Can you work these out from the model? Positions are in its coordinate system, mm. A direction names the side the tool comes from. Give positions to 0.01 mm unless a question says otherwise; leave off trailing zeros. Loops run counter-clockwise (first coordinate to the right, second up) from the corner with the lowest first, then second, coordinate; pieces in that order, holes last.
from build123d import *

# Parameters (mm, degrees)
SKETCH1_R           = 2.794
BOSS_EXTRUDE1_DEPTH = 5.08
SKETCH3_W           = 25.4
SKETCH3_H           = 11.43
BOSS_EXTRUDE2_DEPTH = 45.72
SKETCH4_W           = 22.096687199
SKETCH4_H           = 11.43
BOSS_EXTRUDE3_DEPTH = 12.7
BOSS_EXTRUDE5_DEPTH = 11.43
SKETCH7_W           = 18.793374398
SKETCH7_H           = 33.02
CUT_EXTRUDE3_DEPTH  = 12.7


with BuildPart() as part:
    # Sketch1 → Boss-Extrude1 (new body)
    with BuildSketch(Plane.XY):
        Polygon((-57.15, 2.54), (-57.15, -2.54), (-57.15, -5.715), (57.15, -5.715), (57.15, -2.54), (57.15, 2.54), (57.15, 5.715), (-57.15, 5.715), align=None)
        with Locations((50.8, 0)):
            Circle(SKETCH1_R, mode=Mode.SUBTRACT)
        with Locations((-50.8, 0)):
            Circle(SKETCH1_R, mode=Mode.SUBTRACT)
    extrude(amount=BOSS_EXTRUDE1_DEPTH)

    # Sketch3 → Boss-Extrude2 (add)
    with BuildSketch(Plane.XY.offset(5.08)):
        Rectangle(SKETCH3_W, SKETCH3_H)
    extrude(amount=BOSS_EXTRUDE2_DEPTH)

    # Sketch4 → Boss-Extrude3 (add)
    with BuildSketch(Plane.XY.offset(50.8)):
        with Locations((23.7483436, 0)):
            Rectangle(SKETCH4_W, SKETCH4_H)
        with Locations((-23.7483436, 0)):
            Rectangle(SKETCH4_W, SKETCH4_H)
    extrude(amount=-BOSS_EXTRUDE3_DEPTH)

    # Sketch5 → Boss-Extrude5 (add)
    with BuildSketch(Plane.XZ.offset(5.715)):
        Polygon((-44.45, 5.08), (-12.7, 5.08), (-12.7, 38.1), (-21.519444444, 38.1), align=None)
        Polygon((12.7, 38.1), (12.7, 5.08), (44.45, 5.08), (21.519444444, 38.1), align=None)
    extrude(amount=-BOSS_EXTRUDE5_DEPTH)

    # Sketch7 → Cut-Extrude3 (cut)
    with BuildSketch(Plane.XZ.offset(5.715)):
        with Locations((0, 21.59)):
            Rectangle(SKETCH7_W, SKETCH7_H)
    extrude(amount=-CUT_EXTRUDE3_DEPTH, mode=Mode.SUBTRACT)


solid = part.part
(1) Which directions (+Z, -Z, +X, -X, +Y, -Y) give clear straight access to the entire face, cutting with the end or side of a thin tool? Please do faces 1 (the flat face through (-9.397, 0, 21)), 2 (the flat face through (49, 3, 5.08)), 3 (the flat face through (-32.824, -0.08, 21.821)).
Returned:
face 1: +Y, -Y
face 2: +Z, +X, +Y, -Y
face 3: -X, +Y, -Y
(2) Will these pins go through, and if not, where does the flat tip stop? P1, Ø5.5, axis at x = -52, y = -1, coming from the +Z side; P2, Ø5, axis at x = 12.5, y = -3, coming from the -Z side; P3, Ø3.5, axis at y = -1.5, z = 45.5, coming from the +X side; P4, Ø4, axis at y = 3.5, z = 33, coming from the +X side.
Returned:
P1: stops at z = 5.08
P2: stops at z = 0
P3: stops at x = 34.8
P4: stops at x = 26.45
(3) Suppose I cut it at B-B on y = 0. List the corners of the cut face in (x, z) for me.
Returned:
outline: (-57.15, 0) - (-53.59, 0) - (-53.59, 5.08) - (-57.15, 5.08) - close; (-48.01, 0) - (48.01, 0) - (48.01, 5.08) - (44.45, 5.08) - (21.52, 38.1) - (34.8, 38.1) - (34.8, 50.8) - (-34.8, 50.8) - (-34.8, 38.1) - (-21.52, 38.1) - (-44.45, 5.08) - (-48.01, 5.08) - close; (53.59, 0) - (57.15, 0) - (57.15, 5.08) - (53.59, 5.08) - close; hole (-9.4, 5.08) - (9.4, 5.08) - (9.4, 38.1) - (-9.4, 38.1) - close
(4) Thinking about a two-plate mould opening in X: for faces 4 (the cylindrical face through (48.01, 0.12, 2.5)), 5 (the flat face through (34.797, 0, 45)), 6 (the flat face through (-34.797, 0, 45)), 7 (the flat face through (0, 0, 5.08)), which applies, pulls with the +X half, pulls with the -X half, needs draft (parallel to the pull), parting line crosses it, or undercut?
Returned:
face 4: undercut
face 5: pulls with the +X half
face 6: pulls with the -X half
face 7: undercut
(5) Please list where these lines run through material, in increasing order: probe 1 along Z at (x, y) = (8, 3.25); probe 2 along Y at (x, z) = (-50.8, 3.8) (3 decimals); probe 3 along X at (y, z) = (2, 5).
Returned:
probe 1: z = 0 to 5.08, 38.1 to 50.8
probe 2: y = -5.715 to -2.794, 2.794 to 5.715
probe 3: x = -57.15 to -52.75, -48.85 to 48.85, 52.75 to 57.15
(6) Suppose I cut it at C-C on z = 20. List the corners of the cut face in (x, y) for me (3 decimals), plus the area to 3 significant figures.
Returned:
outline: (-34.089, -5.715) - (-9.397, -5.715) - (-9.397, 5.715) - (-34.089, 5.715) - close; (9.397, -5.715) - (34.089, -5.715) - (34.089, 5.715) - (9.397, 5.715) - close
area: 564 mm2
(7) Suppose I cut it at A-A on x = -50.8. List the corners of the cut face in (y, z) for me (3 decimals), plus the area to 3 significant figures.
Returned:
outline: (-5.715, 0) - (-2.794, 0) - (-2.794, 5.08) - (-5.715, 5.08) - close; (2.794, 0) - (5.715, 0) - (5.715, 5.08) - (2.794, 5.08) - close
area: 29.7 mm2
(8) Suppose I cut it at D-D on x = 41. List the corners of the cut face in (y, z) for me (3 decimals).
Returned:
outline: (-5.715, 0) - (5.715, 0) - (5.715, 10.048) - (-5.715, 10.048) - close
